from build123d import *

# Parameters (mm, degrees)
SKETCH2_W           = 500
SKETCH2_H           = 160
SKETCH2_R           = 15
SKETCH2_R_2         = 5
SKETCH2_R_3         = 3.5
SKETCH2_R_4         = 2
SKETCH2_R_5         = 3.25
BOSS_EXTRUDE1_DEPTH = 6
FILLET1_R           = 5


with BuildPart() as part:
    # Sketch2 → Boss-Extrude1 (new body)
    with BuildSketch(Plane.XY):
        with Locations((50, 0)):
            Rectangle(SKETCH2_W, SKETCH2_H)
        with Locations((50, 0)):
            Circle(SKETCH2_R, mode=Mode.SUBTRACT)
        with Locations((-50, 0)):
            Circle(SKETCH2_R_2, mode=Mode.SUBTRACT)
        with Locations((150, 0)):
            Circle(SKETCH2_R_2, mode=Mode.SUBTRACT)
        with Locations((-159, 20)):
            Circle(SKETCH2_R_3, mode=Mode.SUBTRACT)
        with Locations((-159, -20)):
            Circle(SKETCH2_R_3, mode=Mode.SUBTRACT)
        with Locations((259, -20)):
            Circle(SKETCH2_R_3, mode=Mode.SUBTRACT)
        with Locations((259, 20)):
            Circle(SKETCH2_R_3, mode=Mode.SUBTRACT)
        with Locations((134, 0)):
            Circle(SKETCH2_R_4, mode=Mode.SUBTRACT)
        with Locations((166, 0)):
            Circle(SKETCH2_R_4, mode=Mode.SUBTRACT)
        with Locations((-66, 0)):
            Circle(SKETCH2_R_4, mode=Mode.SUBTRACT)
        with Locations((-34, 0)):
            Circle(SKETCH2_R_4, mode=Mode.SUBTRACT)
        with Locations((66.5, 16.5)):
            Circle(SKETCH2_R_5, mode=Mode.SUBTRACT)
        with Locations((33.5, 16.5)):
            Circle(SKETCH2_R_5, mode=Mode.SUBTRACT)
        with Locations((33.5, -16.5)):
            Circle(SKETCH2_R_5, mode=Mode.SUBTRACT)
        with Locations((66.5, -16.5)):
            Circle(SKETCH2_R_5, mode=Mode.SUBTRACT)
    extrude(amount=BOSS_EXTRUDE1_DEPTH)

    # Fillet1
    fillet1_edges = [part.edges().sort_by_distance(p)[0] for p in [
        (-200, -80, 3),
        (-200, 80, 3),
        (300, 80, 3),
        (300, -80, 3),
    ]]
    fillet(fillet1_edges, radius=FILLET1_R)


solid = part.part
The listing builds one solid part. Answer for the finished solid, in the listing's coordinates (mm). Coordinates: 2 decimals unless noted, no trailing zeros. Write each loop counter-clockwise with the first axis right and the second up, starting at its lowest first coordinate (ties: lowest second). Pieces come first, ordered by that corner, then holes. Notation, with made-up numbers: M -15.5,69.5 L -0.5,69.5 A8 ccw -0.5,80.5 Z; hole C 87,-11.75 d2. An arc over 180 degrees is marked long. Put each result on its own line as item: value. Start each with the question number.
1. Consider line 1 (Y direction, x = 66.5, z = 4.3); line 2 (Y direction, x = 259, z = 0.7); line 3 (Y direction, x = -34, z = 1.75). Determine where each line is inside the solid, lowest interval first. Write a range as from..to.
2. A cutting plane is placed at A-A on x = 150. Write down the section's boundary in (y, z).
3. For a pull along X with two mould halves and no side action, classify faces 1 (the cylindrical face through (145, 0, 3)), 2 (the flat face through (47, 19, 0)) as pulls with the +X half, pulls with the -X half, needs draft (parallel to the pull), parting line crosses it, or undercut.
4. A cutting plane is placed at B-B on z = 3.7. Count the separate pieces of the cut face and the enclosed holes in it, then the cut area to 3 significant figures.
Resolved:
1. line 1: y = -80..-19.75, -13.25..13.25, 19.75..80
1. line 2: y = -80..-23.5, -16.5..16.5, 23.5..80
1. line 3: y = -80..-2, 2..80
2. outline: M -80,0 L -5,0 L -5,6 L -80,6 Z; M 5,0 L 80,0 L 80,6 L 5,6 Z
3. face 1: undercut
3. face 2: needs draft
4. separate pieces: 1
4. enclosed holes: 15
4. area: 78,800 mm2
